The model under review builds one solid part; all positions refer to its coordinate system, in mm. A direction names the side the tool comes from. Round coordinates to 2 decimals unless told otherwise and drop trailing zeros. Write each loop counter-clockwise with the first axis right and the second up, starting at its lowest first coordinate (ties: lowest second). Pieces come first, ordered by that corner, then holes. Notation, with made-up numbers: (32, -4.75) -> (40, -4.75) arc R27 cw to (40, 24.25) -> close; hole circle Ø2 at (-15.75, -22). An arc over 180 degrees is marked (long way). Return JSON: item names as keys, results as strings. Group by question number.
1. Mouldability with a two-part tool opening along X and no side actions: class faces 5 (the flat face through (2.9, 3, 2)), 6 (the flat face through (-5, 25, 2)), 7 (the flat face through (-3, -5, 2)) as pulls with the +X half, pulls with the -X half, needs draft (parallel to the pull), parting line crosses it, or undercut.
2. Take a section at A-A, the plane y = 20. Write out the cut boundary in (x, z).
3. For line 1 along Y through (x, z) = (30.8, 1.9); line 2 along Y through (x, z) = (7.5, 4.25); line 3 along X through (y, z) = (36, 3.5), list the stretches that pass through material, from the lowest coordinate up. Write a range as from..to.
4. Tool access review of faces 1 (the flat face through (64, 50, 2)), 2 (the flat face through (20, -2, 2)), 3 (the flat face through (33, 55, 2)), 4 (the flat face through (63.5, 8, 2)): name each direction out of +Z, -Z, +X, -X, +Y, -Y from which nothing blocks a thin tool from reaching the whole face with its end or side.
5. Take a section at C-C, the plane y = 6. Write out the cut boundary in (x, z).
6. Take a section at B-B, the plane x = 30.8. Write out the cut boundary in (y, z), then the cut area to 3 significant figures.
7. Clearance check with flat-ended pins moving along their axes: P1, Ø1.3, axis at x = 59.5, z = 2, coming from the +Y side; P2, Ø4.5, axis at x = 30.8, y = 6, coming from the -Z side; P3, Ø1.5, axis at x = 14, z = 3.5, coming from the -Y side. State where each tip first meets the part, or that it passes through.
8. Take a section at D-D, the plane z = 0.75. Give the number of separate pieces and of enclosed holes in the cut face, then the cut area to 3 significant figures.
from build123d import *

# Parameters (mm, degrees)
BOSS_EXTRUDE1_DEPTH = 5
SKETCH2_R           = 2
CUT_EXTRUDE2_DEPTH  = 5


with BuildPart() as part:
    # Sketch1 → Boss-Extrude1 (new body)
    with BuildSketch(Plane.XY):
        Polygon((2.9, 50), (0, 50), (0, 55), (-5, 55), (-5, -5), (0, -5), (0, 0), (2.9, 0), (2.9, 6.8), (1.5, 6.8), (1.5, 10), (2.9, 10), (2.9, 17), (7.1, 17), (7.1, 10), (8.5, 10), (8.5, 6.8), (7.1, 6.8), (7.1, 0), (20, 0), (20, -5), (45, -5), (45, 0), (57.9, 0), (57.9, 6.8), (56.5, 6.8), (56.5, 10), (57.9, 10), (57.9, 17), (62.1, 17), (62.1, 10), (63.5, 10), (63.5, 6.8), (62.1, 6.8), (62.1, 0), (65, 0), (65, -5), (70, -5), (70, 55), (65, 55), (65, 50), (62.1, 50), (62.1, 43.2), (63.5, 43.2), (63.5, 40), (62.1, 40), (62.1, 33), (57.9, 33), (57.9, 40), (56.5, 40), (56.5, 43.2), (57.9, 43.2), (57.9, 50), (45, 50), (45, 55), (20, 55), (20, 50), (7.1, 50), (7.1, 43.2), (8.5, 43.2), (8.5, 40), (7.1, 40), (7.1, 33), (2.9, 33), (2.9, 40), (1.5, 40), (1.5, 43.2), (2.9, 43.2), align=None)
    extrude(amount=BOSS_EXTRUDE1_DEPTH)

    # Sketch2 → Cut-Extrude2 (cut)
    with BuildSketch(Plane(origin=(0, 0, 0), x_dir=(-1, 0, 0), z_dir=(0, 0, -1))):
        with Locations((-46.3, 20)):
            Circle(SKETCH2_R)
        with Locations((-46.3, 6)):
            Circle(SKETCH2_R)
        with Locations((-30.8, 6)):
            Circle(SKETCH2_R)
        with Locations((-30.8, 20)):
            Circle(SKETCH2_R)
    extrude(amount=-CUT_EXTRUDE2_DEPTH, mode=Mode.SUBTRACT)


solid = part.part
Output:
{
 "1": {"face 5": "undercut", "face 6": "pulls with the -X half", "face 7": "needs draft"},
 "2": {"outline": "(-5, 0) -> (28.8, 0) -> (28.8, 5) -> (-5, 5) -> close; (32.8, 0) -> (44.3, 0) -> (44.3, 5) -> (32.8, 5) -> close; (48.3, 0) -> (70, 0) -> (70, 5) -> (48.3, 5) -> close"},
 "3": {"line 1": "y = -5..4, 8..18, 22..55", "line 2": "y = 0..6.8, 10..40, 43.2..50", "line 3": "x = -5..2.9, 7.1..57.9, 62.1..70"},
 "4": {"face 1": "+Z, -Z, +Y", "face 2": "+Z, -Z, -Y", "face 3": "+Z, -Z, +X, -X, +Y", "face 4": "+Z, -Z"},
 "5": {"outline": "(-5, 0) -> (2.9, 0) -> (2.9, 5) -> (-5, 5) -> close; (7.1, 0) -> (28.8, 0) -> (28.8, 5) -> (7.1, 5) -> close; (32.8, 0) -> (44.3, 0) -> (44.3, 5) -> (32.8, 5) -> close; (48.3, 0) -> (57.9, 0) -> (57.9, 5) -> (48.3, 5) -> close; (62.1, 0) -> (70, 0) -> (70, 5) -> (62.1, 5) -> close"},
 "6": {"outline": "(-5, 0) -> (4, 0) -> (4, 5) -> (-5, 5) -> close; (8, 0) -> (18, 0) -> (18, 5) -> (8, 5) -> close; (22, 0) -> (55, 0) -> (55, 5) -> (22, 5) -> close", "area": "260 mm^2"},
 "7": {"P1": "stops at y = 33", "P2": "stops at z = 0", "P3": "stops at y = 0"},
 "8": {"separate pieces": "1", "enclosed holes": "4", "area": "3,730 mm^2"}
}
